The listing builds one solid part. Answer for the finished solid, in the listing's coordinates (mm). Face numbers are marked on the shaded views. A direction names the side the tool comes from. Round coordinates to 2 decimals unless told otherwise and drop trailing zeros. Write each loop counter-clockwise with the first axis right and the second up, starting at its lowest first coordinate (ties: lowest second). Pieces come first, ordered by that corner, then holes.
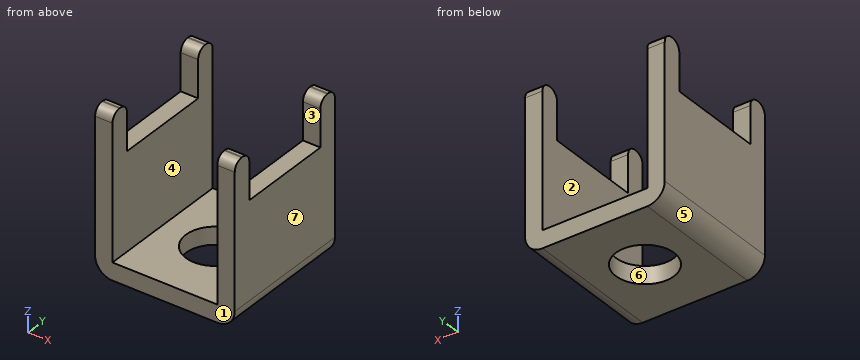
from build123d import *

# Parameters (mm, degrees)
BOSS_EXTRUDE1_DEPTH = 11.7
CUT_EXTRUDE2_REACH  = 23.71
SKETCH2_W           = 4
SKETCH2_H           = 8.3
FILLET1_R           = 0.8
SKETCH3_R           = 2.5
CUT_EXTRUDE3_DEPTH  = 1.5


with BuildPart() as part:
    # Sketch1 → Boss-Extrude1 (new body)
    with BuildSketch(Plane(origin=(0, 0, 0), x_dir=(1, 0, 0), z_dir=(0, 1, 0))):
        with BuildLine():
            Line((0, 0), (-1.5, 0))
            Line((-1.5, 0), (-1.5, 12.3))
            ThreePointArc((-1.5, 12.3), (-1.060660172, 13.360660172), (0, 13.8))
            Line((0, 13.8), (9, 13.8))
            ThreePointArc((9, 13.8), (10.060660172, 13.360660172), (10.5, 12.3))
            Line((10.5, 12.3), (10.5, 0))
            Line((10.5, 0), (9, 0))
            Line((9, 0), (9, 12.3))
            Line((9, 12.3), (0, 12.3))
            Line((0, 12.3), (0, 0))
        make_face()
    extrude(amount=BOSS_EXTRUDE1_DEPTH)

    # Cut-Extrude2: up to this face of the body (flat: up to its plane)
    cut_extrude2_end = Plane(part.part.faces().sort_by_distance((-1.5, 5.85, -6.15))[0])
    # Sketch2 → Cut-Extrude2 (cut, up to the picked face)
    with BuildSketch(Plane(origin=(10.5, 0, 0), x_dir=(0, 0, -1), z_dir=(1, 0, 0)), mode=Mode.PRIVATE) as cut_extrude2_sk1:
        with Locations((2, 5.85)):
            Rectangle(SKETCH2_W, SKETCH2_H)
    cut_extrude2_tool1 = split(extrude(cut_extrude2_sk1.sketch, amount=-CUT_EXTRUDE2_REACH, mode=Mode.PRIVATE), bisect_by=cut_extrude2_end, keep=Keep.BOTH, mode=Mode.PRIVATE)
    add(cut_extrude2_tool1.solids().sort_by(Axis((10.5, 5.85, -2), (-1, 0, 0)))[0], mode=Mode.SUBTRACT)

    # Fillet1
    fillet1_edges = [part.edges().sort_by_distance(p)[0] for p in [
        (-0.75, 0, 0),
        (9.75, 0, 0),
        (9.75, 11.7, 0),
        (-0.75, 1.7, 0),
        (9.75, 1.7, 0),
        (-0.75, 11.7, 0),
        (-0.75, 10, 0),
        (9.75, 10, 0),
    ]]
    fillet(fillet1_edges, radius=FILLET1_R)

    # Sketch3 → Cut-Extrude3 (cut)
    with BuildSketch(Plane(origin=(0, 0, -13.8), x_dir=(-1, 0, 0), z_dir=(0, 0, -1))):
        with Locations((-4.5, 5.85)):
            Circle(SKETCH3_R)
    extrude(amount=-CUT_EXTRUDE3_DEPTH, mode=Mode.SUBTRACT)


solid = part.part
1. Straight lines are drawn through the part: line 1 along Y through (x, z) = (4.5, -13.5); line 2 along X through (y, z) = (1.75, -5); line 3 along Z through (x, y) = (7.5, 7). For each, find the intervals that lie inside material, in ascending order.
Geometry says:
line 1: y = 0 to 3.35, 8.35 to 11.7
line 2: x = -1.5 to 0, 9 to 10.5
line 3: z = -13.8 to -12.3
2. Section A-A on z = -3.75 is taken. Determine the outline of the cut face in (x, y).
Geometry says:
outline: (-1.5, 0) - (0, 0) - (0, 1.7) - (-1.5, 1.7) - close; (-1.5, 10) - (0, 10) - (0, 11.7) - (-1.5, 11.7) - close; (9, 0) - (10.5, 0) - (10.5, 1.7) - (9, 1.7) - close; (9, 10) - (10.5, 10) - (10.5, 11.7) - (9, 11.7) - close
3. Section B-B on x = 4.5 is taken. Determine the outline of the cut face in (y, z).
Geometry says:
outline: (0, -13.8) - (3.35, -13.8) - (3.35, -12.3) - (0, -12.3) - close; (8.35, -13.8) - (11.7, -13.8) - (11.7, -12.3) - (8.35, -12.3) - close
4. For a pull along X with two mould halves and no side action, classify the marked faces 4, 5, 6 and 7 as released by +X, released by -X, zero draft, split by the parting line, or undercut.
Geometry says:
face 4: undercut
face 5: released by -X
face 6: undercut
face 7: released by +X
5. Section C-C on y = 7.25 is taken. Determine the outline of the cut face in (x, z), plus the area to 3 significant figures.
Geometry says:
outline: (-1.5, -12.3) arc R1.5 ccw to (0, -13.8) - (2.43, -13.8) - (2.43, -12.3) - (0, -12.3) - (0, -4) - (-1.5, -4) - close; (6.57, -13.8) - (9, -13.8) arc R1.5 ccw to (10.5, -12.3) - (10.5, -4) - (9, -4) - (9, -12.3) - (6.57, -12.3) - close
area: 35.7 mm2
6. A tool of negligible diameter and unlimited length cuts with its end or side. For the marked faces 1, 2 and 3, from which of +Z, -Z, +X, -X, +Y, -Y can it reach the whole face along a straight path? Write none if from no direction.
Geometry says:
face 1: +Z, -Z, +X, -X, -Y
face 2: +Z, +Y, -Y
face 3: +Z, +X, -X
7. Section D-D on y = 9 is taken. Determine the outline of the cut face in (x, z), plus the area to 3 significant figures.
Geometry says:
outline: (-1.5, -12.3) arc R1.5 ccw to (0, -13.8) - (9, -13.8) arc R1.5 ccw to (10.5, -12.3) - (10.5, -4) - (9, -4) - (9, -12.3) - (0, -12.3) - (0, -4) - (-1.5, -4) - close
area: 41.9 mm2
8. Given pin 1 (1.2 mm diameter, centred on x = -1, y = 4.5, fed in from +Z); pin 2 (4 mm diameter, centred on x = 3.5, y = 7, fed in from -Z); pin 3 (2 mm diameter, centred on x = 3.5, y = 10, fed in from +Z), each flat-ended and moving along its own axis, determine where each tip first touches the part or whether it passes through.
Geometry says:
pin 1: stops at z = -4
pin 2: stops at z = -13.8
pin 3: stops at z = -12.3
